from build123d import *

# Parameters (mm, degrees)
BOSS_EXTRUDE1_DEPTH   = 1
F_6_CLEARANCE_HOLE1_D = 3.7973


with BuildPart() as part:
    # Sketch1 → Boss-Extrude1 (new body)
    # profile 1 of 3: a face of its own
    with BuildSketch(Plane(origin=(0, 0, 0), x_dir=(1, 0, 0), z_dir=(0, 1, 0))):
        with BuildLine():
            Line((0.660254038, 5), (-8, 5))
            ThreePointArc((-8, 5), (-13, 0), (-8, -5))
            Line((-8, -5), (2, -5))
            ThreePointArc((2, -5), (-2.829629131, -1.294095226), (-0.5, 4.330127019))
            Line((-0.5, 4.330127019), (0.660254038, 5))
        make_face()
    # profile 2 of 3: a face of its own
    with BuildSketch(Plane(origin=(0, 0, 0), x_dir=(1, 0, 0), z_dir=(0, 1, 0))):
        with BuildLine():
            Line((2, 5), (0.660254038, 5))
            Line((0.660254038, 5), (-0.5, 4.330127019))
            ThreePointArc((-0.5, 4.330127019), (-2.829629131, -1.294095226), (2, -5))
            ThreePointArc((2, -5), (3.294095226, -4.829629131), (4.5, -4.330127019))
            ThreePointArc((4.5, -4.330127019), (6.829629131, 1.294095226), (2, 5))
        make_face()
    # profile 3 of 3: a face of its own
    with BuildSketch(Plane(origin=(0, 0, 0), x_dir=(1, 0, 0), z_dir=(0, 1, 0))):
        with BuildLine():
            Line((10.325317547, 10.580127019), (0.660254038, 5))
            Line((0.660254038, 5), (2, 5))
            ThreePointArc((2, 5), (6.829629131, 1.294095226), (4.5, -4.330127019))
            Line((4.5, -4.330127019), (15.325317547, 1.919872981))
            ThreePointArc((15.325317547, 1.919872981), (17.155444566, 8.75), (10.325317547, 10.580127019))
        make_face()
        with BuildLine():
            ThreePointArc((12.909292144, 4.104551733), (10.313843876, 4.8), (11.009292144, 7.395448267))
            Line((11.009292144, 7.395448267), (12.308330249, 8.145448267))
            ThreePointArc((12.308330249, 8.145448267), (14.903778516, 7.45), (14.208330249, 4.854551733))
            Line((14.208330249, 4.854551733), (12.909292144, 4.104551733))
        make_face(mode=Mode.SUBTRACT)
    extrude(amount=BOSS_EXTRUDE1_DEPTH)

    # #6 Clearance Hole1 (through all)
    with Locations(Plane(origin=(0, 1, 0), x_dir=(1, 0, 0), z_dir=(0, 1, 0))):
        with Locations((-8, 0)):
            Hole(F_6_CLEARANCE_HOLE1_D / 2)


solid = part.part
Can you work these out from the model? Positions are in its coordinate system, mm. A direction names the side the tool comes from. Round coordinates to 2 decimals unless told otherwise and drop trailing zeros. Write each loop counter-clockwise with the first axis right and the second up, starting at its lowest first coordinate (ties: lowest second). Pieces come first, ordered by that corner, then holes. Notation, with made-up numbers: (48.5, 70.25) - (99.5, 70.25) arc R16 cw to (99.5, 76.25) - close; hole circle Ø4 at (-16.5, 18). An arc over 180 degrees is marked (long way). Write each question's results on one line, items separated by ' | '. Start each with the question number.
1) Suppose I cut it at A-A (z = -5.75). List the corners of the cut face in (x, y) for me, and give its area (3 significant figures).
2) Suppose I cut it at B-B (y = 0.7). List the corners of the cut face in (x, z) for me, and give its area (3 significant figures).
3) We'd pull the mould along Z, two halves only. Please class faces 1 (the cylindrical face through (3.276, 0.493, 4.834)), 2 (the cylindrical face through (-13, 0.5, -0.1)), 3 (the cylindrical face through (14.88, 0.49, -7.49)): released by +Z, released by -Z, zero draft, split by the parting line, or undercut.
4) Suppose I cut it at C-C (z = 0.75). List the corners of the cut face in (x, y) for me, and give its area (3 significant figures).
5) Please list where these lines run through material, in increasing order: line 1 (Z direction, x = -8, y = 0.6); line 2 (Z direction, x = -3, y = 0.1); line 3 (Z direction, x = -6.5, y = 0.95).
6) For pin 1 Ø6 at (x, z) = (-8, 0) entering from +Y, with a flat end and sliding along its axis, tell me the tip position at first contact or that it passes through.
7) Suppose I cut it at D-D (x = 6). List the corners of the cut face in (y, z) for me.
8) Which directions (+Z, -Z, +X, -X, +Y, -Y) give clear straight access to the entire face, cutting with the end or side of a thin tool? Please do faces 4 (the flat face through (-3.6, 0.5, -5)), 5 (the flat face through (-3.1, 0.5, 5)), 6 (the flat face through (11.65, 0.493, -7.765)).
Here are the results:
1) outline: (1.96, 0) - (10.06, 0) - (10.06, 1) - (1.96, 1) - close; (15, 0) - (17.8, 0) - (17.8, 1) - (15, 1) - close | area: 10.9 mm2
2) outline: (-8, -5) - (0.66, -5) - (10.33, -10.58) arc R5 ccw to (15.33, -1.92) - (4.5, 4.33) arc R5 ccw to (2, 5) - (-8, 5) arc R5 ccw to start; hole circle Ø3.8 at (-8, 0); hole (11.01, -7.4) - (12.31, -8.15) arc R1.9 ccw to (14.21, -4.85) - (12.91, -4.1) arc R1.9 ccw to start | area: 275 mm2
3) face 1: released by +Z | face 2: split by the parting line | face 3: undercut
4) outline: (-12.94, 0) - (-9.74, 0) - (-9.74, 1) - (-12.94, 1) - close; (-6.26, 0) - (10.7, 0) - (10.7, 1) - (-6.26, 1) - close | area: 20.2 mm2
5) line 1: z = -5 to -1.9, 1.9 to 5 | line 2: z = -5 to 5 | line 3: z = -5 to -1.16, 1.16 to 5
6) pin 1: stops at y = 1
7) outline: (0, -8.08) - (1, -8.08) - (1, 3.46) - (0, 3.46) - close
8) face 4: -Z, -X, +Y, -Y | face 5: +Z, +X, -X, +Y, -Y | face 6: +Y, -Y
